```python
from build123d import *

# Parameters (mm, degrees)
SKETCH11_R          = 82.5
SKETCH11_R_2        = 20
BOSS_EXTRUDE7_DEPTH = 10
SKETCH11_9_R        = 82.5
SKETCH11_9_R_2      = 80
BOSS_EXTRUDE8_DEPTH = 70
SKETCH11_10_R       = 65
SKETCH11_10_R_2     = 62.5
BOSS_EXTRUDE9_DEPTH = 42.5
FILLET2_R           = 3
FILLET3_R           = 3


with BuildPart() as part:
    # Sketch11 → Boss-Extrude7 (new body)
    with BuildSketch(Plane(origin=(0, 0, 0), x_dir=(1, 0, 0), z_dir=(0, 1, 0))):
        with Locations(Location((0, 0, 0), (0, 0, 270))):
            Circle(SKETCH11_R)
        with Locations(Location((0, 0, 0), (0, 0, 270))):
            Circle(SKETCH11_R_2, mode=Mode.SUBTRACT)
    extrude(amount=BOSS_EXTRUDE7_DEPTH)

    # Sketch11_9 → Boss-Extrude8 (add)
    with BuildSketch(Plane(origin=(0, 0, 0), x_dir=(1, 0, 0), z_dir=(0, 1, 0))):
        with Locations(Location((0, 0, 0), (0, 0, 270))):
            Circle(SKETCH11_9_R)
        with Locations(Location((0, 0, 0), (0, 0, 270))):
            Circle(SKETCH11_9_R_2, mode=Mode.SUBTRACT)
    extrude(amount=BOSS_EXTRUDE8_DEPTH)

    # Sketch11_10 → Boss-Extrude9 (add)
    with BuildSketch(Plane(origin=(0, 0, 0), x_dir=(1, 0, 0), z_dir=(0, 1, 0))):
        with Locations(Location((0, 0, 0), (0, 0, 270))):
            Circle(SKETCH11_10_R)
        with Locations(Location((0, 0, 0), (0, 0, 270))):
            Circle(SKETCH11_10_R_2, mode=Mode.SUBTRACT)
    extrude(amount=BOSS_EXTRUDE9_DEPTH)

    # Fillet2
    fillet2_edges = [part.edges().sort_by_distance(p)[0] for p in [
        (0, 10, -80),
    ]]
    fillet(fillet2_edges, radius=FILLET2_R)

    # Fillet3
    fillet3_edges = [part.edges().sort_by_distance(p)[0] for p in [
        (0, 10, -65),
    ]]
    fillet(fillet3_edges, radius=FILLET3_R)


solid = part.part
```
Read the model definition and answer for the solid it produces. Units are mm, in the model's axes. A direction names the side the tool comes from. Give positions to 0.01 mm unless a question says otherwise; leave off trailing zeros. Write each loop counter-clockwise with the first axis right and the second up, starting at its lowest first coordinate (ties: lowest second). Pieces come first, ordered by that corner, then holes. Notation, with made-up numbers: M 57.25,86.25 L 61.25,86.25 A19 ccw 61.25,115.25 Z; hole C 47.5,4.25 d7. An arc over 180 degrees is marked long. Put each result on its own line as item: value. Start each with the question number.
1. The part is cut by section A-A, the plane x = 0. Give the vertices of the cut face in (y, z), and give its area (3 significant figures).
2. The part is cut by section B-B, the plane z = 0. Give the vertices of the cut face in (x, y), and give its area (3 significant figures).
3. Each of these flat-tipped pins is pushed along its axis until it touches: pin 1 Ø8 at (y, z) = (39.5, 18.5) entering from +X; pin 2 Ø1.5 at (y, z) = (35.5, 38) entering from +X; pin 3 Ø2 at (y, z) = (57.5, -13) entering from -X. Where does it stop, or does it pass through?
4. Consider line 1 along X through (y, z) = (19, 0); line 2 along X through (y, z) = (3, 0); line 3 along X through (y, z) = (55.5, 0). Determine where each line is inside the solid, lowest interval first.
5. For a pull along X with two mould halves and no side action, classify faces 1 (the cylindrical face through (19.52, 27.54, 62)), 2 (the flat face through (-17, 0, 17)), 3 (the cylindrical face through (2.75, 26.02, -62.44)), 4 (the cylindrical face through (-80.54, 34.51, -17.88)) as released by +X, released by -X, zero draft, split by the parting line, or undercut.
6. Which of the six approach directions +Z, -Z, +X, -X, +Y, -Y give full straight-line access (tool end or side, diameter ignored) to faces 5 (the flat face through (-68, 10, 5)), 6 (the cylindrical face through (-19.524, 4.93, -4.336))?
7. The part is cut by section C-C, the plane y = 17. Give the vertices of the cut face in (x, z), and give its area (3 significant figures).
Final values:
1. outline: M 0,-82.5 L 70,-82.5 L 70,-80 L 13,-80 A3 cw 10,-77 L 10,-68 A3 cw 13,-65 L 42.5,-65 L 42.5,-62.5 L 10,-62.5 L 10,-20 L 0,-20 Z; M 0,20 L 10,20 L 10,62.5 L 42.5,62.5 L 42.5,65 L 13,65 A3 cw 10,68 L 10,77 A3 cw 13,80 L 70,80 L 70,82.5 L 0,82.5 Z
1. area: 1,720 mm²
2. outline: M -82.5,0 L -20,0 L -20,10 L -62.5,10 L -62.5,42.5 L -65,42.5 L -65,13 A3 cw -68,10 L -77,10 A3 cw -80,13 L -80,70 L -82.5,70 Z; M 20,0 L 82.5,0 L 82.5,70 L 80,70 L 80,13 A3 cw 77,10 L 68,10 A3 cw 65,13 L 65,42.5 L 62.5,42.5 L 62.5,10 L 20,10 Z
2. area: 1,720 mm²
3. pin 1: stops at x = 81.22
3. pin 2: stops at x = 73.61
3. pin 3: stops at x = -81.62
4. line 1: x = -82.5 to -80, -65 to -62.5, 62.5 to 65, 80 to 82.5
4. line 2: x = -82.5 to -20, 20 to 82.5
4. line 3: x = -82.5 to -80, 80 to 82.5
5. face 1: undercut
5. face 2: zero draft
5. face 3: undercut
5. face 4: split by the parting line
6. face 5: +Y
6. face 6: +Y, -Y
7. outline: C 0,0 d165; C 0,0 d130; hole C 0,0 d160; hole C 0,0 d125
7. area: 2,280 mm²
